from build123d import *

# Parameters (mm, degrees)
F0_W      = 356
F0_H      = 50
F1_DEPTH  = 5
F2_R      = 5
F2_R_2    = 12.5
F3_DEPTH  = 5.001
F4_R      = 1.5
F5_DEPTH  = 5.001
F6_W      = 49.406879
F6_H      = 21.095738
F7_DEPTH  = 25
F9_W      = 63.062
F9_H      = 50
F10_DEPTH = 5
F11_R     = 3
F12_DEPTH = 25


with BuildPart() as f1:
    # F0 (on Top) → F1 (new body)
    with BuildSketch(Plane.XY):
        Rectangle(F0_W, F0_H)
    extrude(amount=F1_DEPTH)

    # F2 (on face) → F3 (cut, through all)
    with BuildSketch(Plane.XY.offset(5)):
        with Locations((-155, 12.335402)):
            Circle(F2_R)
        with Locations((155, 12.335402)):
            Circle(F2_R)
        with Locations((-48.086096, 0)):
            Circle(F2_R_2)
        with Locations((51.913904, 0)):
            Circle(F2_R_2)
    extrude(amount=-F3_DEPTH, mode=Mode.SUBTRACT)

    # F4 (on face) → F5 (cut, through all)
    with BuildSketch(Plane.XY.offset(5)):
        with Locations((0, 2.148001)):
            Circle(F4_R)
        with Locations((100, 2.148001)):
            Circle(F4_R)
        with Locations((-100, 2.148001)):
            Circle(F4_R)
    extrude(amount=-F5_DEPTH, mode=Mode.SUBTRACT)

    # F9 (on Top) → F10 (join, through all)
    with BuildSketch(Plane.XY):
        with Locations((-209.531, 0)):
            Rectangle(F9_W, F9_H)
    extrude(amount=F10_DEPTH)

    # F11 (on face) → F12 (cut)
    with BuildSketch(Plane.XY.offset(5)):
        with Locations((-223.56236, 5)):
            Circle(F11_R)
        with Locations((-223.56236, -15)):
            Circle(F11_R)
    extrude(amount=-F12_DEPTH, mode=Mode.SUBTRACT)


with BuildPart() as f7:
    # F6 (on Top) → F7 (new body)
    with BuildSketch(Plane.XY):
        with Locations((37.024449, 48.380569)):
            Rectangle(F6_W, F6_H)
    extrude(amount=F7_DEPTH)


solid = f1.part
For this review, take the finished solid that the model builds, in its own axes (mm). Round coordinates to 2 decimals unless told otherwise and drop trailing zeros. Write each loop counter-clockwise with the first axis right and the second up, starting at its lowest first coordinate (ties: lowest second). Pieces come first, ordered by that corner, then holes. Notation, with made-up numbers: (44.25, 66) -> (62.25, 66) arc R10 ccw to (62.25, 71) -> close; hole circle Ø6 at (32, 21.5). An arc over 180 degrees is marked (long way). Use CSV: the item, a comma, the result in double quotes.
(1) Consider section A-A, the plane x = -155. Give the boundary of the cut face in (y, z).
Computed values:
outline,"(-25, 0) -> (7.34, 0) -> (7.34, 5) -> (-25, 5) -> close; (17.34, 0) -> (25, 0) -> (25, 5) -> (17.34, 5) -> close"
(2) Consider section B-B, the plane z = 2.1. Give the number of separate pieces and of enclosed holes in the cut face, plus the area to 3 significant figures.
Computed values:
separate pieces,"1"
enclosed holes,"9"
area,"19,700 mm²"
(3) Draft analysis for pull direction X (two halves, no side actions). For faces 1 (the face through (-34, 0, 0)), 2 (the face through (-58.006, -7.606, 2.535)), state which applies: +X half, -X half, draft (parallel to the pull), parting line (faces both ways), or undercut.
Computed values:
face 1,"draft"
face 2,"undercut"
(4) To check wall thickness, follow L1, parallel to X at y = 13, z = 0.7; L2, parallel to Y at x = -155, z = 3.45; L3, parallel to Y at x = 100, z = 1.1. State the ranges of each line that lie inside material, in increasing order. Write a range as [from, to].
Computed values:
L1,"[-241.06, -159.96], [-150.04, 150.04], [159.96, 178]"
L2,"[-25, 7.34], [17.34, 25]"
L3,"[-25, 0.65], [3.65, 25]"
(5) Consider section C-C, the plane x = 43.5. Give the boundary of the cut face in (y, z), plus the area to 3 significant figures.
Computed values:
outline,"(-25, 0) -> (-9.24, 0) -> (-9.24, 5) -> (-25, 5) -> close; (9.24, 0) -> (25, 0) -> (25, 5) -> (9.24, 5) -> close"
area,"158 mm²"
